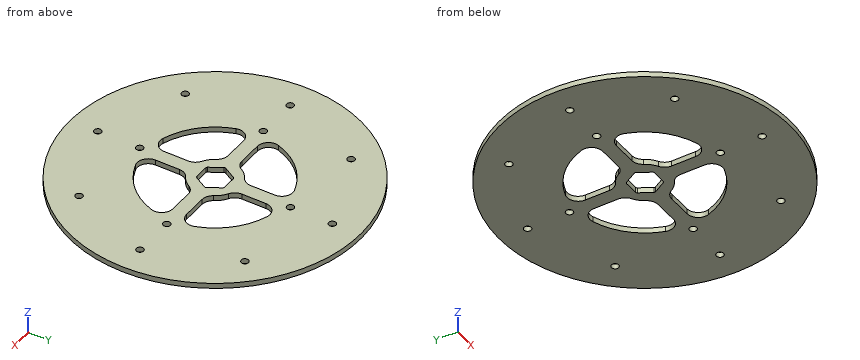
```python
from build123d import *

# Parameters (mm, degrees)
SKETCH1_R           = 66.548
SKETCH1_R_2         = 1.651
BOSS_EXTRUDE1_DEPTH = 2.4384
FILLET6_R           = 0.762


with BuildPart() as part:
    # Sketch1 → Boss-Extrude1 (new body)
    with BuildSketch(Plane.XY):
        Circle(SKETCH1_R)
        with Locations((0, 53.848)):
            Circle(SKETCH1_R_2, mode=Mode.SUBTRACT)
        with Locations((0, 34.619591715)):
            Circle(SKETCH1_R_2, mode=Mode.SUBTRACT)
        with Locations((34.619591715, 0)):
            Circle(SKETCH1_R_2, mode=Mode.SUBTRACT)
        with Locations((0, -34.619591715)):
            Circle(SKETCH1_R_2, mode=Mode.SUBTRACT)
        with Locations((-34.619591715, 0)):
            Circle(SKETCH1_R_2, mode=Mode.SUBTRACT)
        with Locations((38.076285953, 38.076285953)):
            Circle(SKETCH1_R_2, mode=Mode.SUBTRACT)
        with Locations((53.848, 0)):
            Circle(SKETCH1_R_2, mode=Mode.SUBTRACT)
        with Locations((38.076285953, -38.076285953)):
            Circle(SKETCH1_R_2, mode=Mode.SUBTRACT)
        with Locations((0, -53.848)):
            Circle(SKETCH1_R_2, mode=Mode.SUBTRACT)
        with Locations((-38.076285953, -38.076285953)):
            Circle(SKETCH1_R_2, mode=Mode.SUBTRACT)
        with Locations((-53.848, 0)):
            Circle(SKETCH1_R_2, mode=Mode.SUBTRACT)
        with Locations((-38.076285953, 38.076285953)):
            Circle(SKETCH1_R_2, mode=Mode.SUBTRACT)
        with BuildLine():
            Line((25.360281446, 3.175), (14.298079416, 3.175))
            ThreePointArc((14.298079416, 3.175), (11.758079416, 3.855590949), (9.898670365, 5.715))
            ThreePointArc((9.898670365, 5.715), (8.082230509, 8.082230509), (5.715, 9.898670365))
            ThreePointArc((5.715, 9.898670365), (3.855590949, 11.758079416), (3.175, 14.298079416))
            Line((3.175, 14.298079416), (3.175, 25.360281446))
            ThreePointArc((3.175, 25.360281446), (5.270146171, 29.470883302), (9.827380952, 30.190811245))
            ThreePointArc((9.827380952, 30.190811245), (22.450640303, 22.450640303), (30.190811245, 9.827380952))
            ThreePointArc((30.190811245, 9.827380952), (29.470883302, 5.270146171), (25.360281446, 3.175))
        make_face(mode=Mode.SUBTRACT)
        with BuildLine():
            Line((-3.175, 25.360281446), (-3.175, 14.298079416))
            ThreePointArc((-3.175, 14.298079416), (-3.855590949, 11.758079416), (-5.715, 9.898670365))
            ThreePointArc((-5.715, 9.898670365), (-8.082230509, 8.082230509), (-9.898670365, 5.715))
            ThreePointArc((-9.898670365, 5.715), (-11.758079416, 3.855590949), (-14.298079416, 3.175))
            Line((-14.298079416, 3.175), (-25.360281446, 3.175))
            ThreePointArc((-25.360281446, 3.175), (-29.470883302, 5.270146171), (-30.190811245, 9.827380952))
            ThreePointArc((-30.190811245, 9.827380952), (-22.450640303, 22.450640303), (-9.827380952, 30.190811245))
            ThreePointArc((-9.827380952, 30.190811245), (-5.270146171, 29.470883302), (-3.175, 25.360281446))
        make_face(mode=Mode.SUBTRACT)
        with BuildLine():
            Line((3.175, -25.360281446), (3.175, -14.298079416))
            ThreePointArc((3.175, -14.298079416), (3.855590949, -11.758079416), (5.715, -9.898670365))
            ThreePointArc((5.715, -9.898670365), (8.082230509, -8.082230509), (9.898670365, -5.715))
            ThreePointArc((9.898670365, -5.715), (11.758079416, -3.855590949), (14.298079416, -3.175))
            Line((14.298079416, -3.175), (25.360281446, -3.175))
            ThreePointArc((25.360281446, -3.175), (29.470883302, -5.270146171), (30.190811245, -9.827380952))
            ThreePointArc((30.190811245, -9.827380952), (22.450640303, -22.450640303), (9.827380952, -30.190811245))
            ThreePointArc((9.827380952, -30.190811245), (5.270146171, -29.470883302), (3.175, -25.360281446))
        make_face(mode=Mode.SUBTRACT)
        Polygon((7.332348419, 0), (3.666174209, 6.35), (-3.666174209, 6.35), (-7.332348419, 0), (-3.666174209, -6.35), (3.666174209, -6.35), align=None, mode=Mode.SUBTRACT)
        with BuildLine():
            Line((-25.360281446, -3.175), (-14.298079416, -3.175))
            ThreePointArc((-14.298079416, -3.175), (-11.758079416, -3.855590949), (-9.898670365, -5.715))
            ThreePointArc((-9.898670365, -5.715), (-8.082230509, -8.082230509), (-5.715, -9.898670365))
            ThreePointArc((-5.715, -9.898670365), (-3.855590949, -11.758079416), (-3.175, -14.298079416))
            Line((-3.175, -14.298079416), (-3.175, -25.360281446))
            ThreePointArc((-3.175, -25.360281446), (-5.270146171, -29.470883302), (-9.827380952, -30.190811245))
            ThreePointArc((-9.827380952, -30.190811245), (-22.450640303, -22.450640303), (-30.190811245, -9.827380952))
            ThreePointArc((-30.190811245, -9.827380952), (-29.470883302, -5.270146171), (-25.360281446, -3.175))
        make_face(mode=Mode.SUBTRACT)
    extrude(amount=BOSS_EXTRUDE1_DEPTH)

    # Fillet6
    fillet6_edges = [part.edges().sort_by_distance(p)[0] for p in [
        (3.666174209, -6.35, 1.2192),
        (7.332348419, 0, 1.2192),
        (3.666174209, 6.35, 1.2192),
        (-3.666174209, 6.35, 1.2192),
        (-7.332348419, 0, 1.2192),
        (-3.666174209, -6.35, 1.2192),
    ]]
    fillet(fillet6_edges, radius=FILLET6_R)


solid = part.part
```
CAD build for the part. Positions are in the model's coordinates, mm. Give positions to 0.01 mm unless a question says otherwise; leave off trailing zeros. Order: outer loops, then holes, each group sorted by start corner. A loop starts at its lowest first (then second) coordinate and runs counter-clockwise, first axis right, second up. Notation, with made-up numbers: M 17.25,35.25 L 34.25,35.25 A17 ccw 34.25,40.25 Z; hole C -23.75,5.5 d8. An arc over 180 degrees is marked long. Put each result on its own line as item: value. Start each with the question number.
(1) Saw through at A-A, the plane x = 0. Write the cut outline in (y, z), then the cut area to 3 significant figures.
(2) Drill centre lines: line 1 along Y through (x, z) = (0, 1); line 2 along Y through (x, z) = (10, 2.15); line 3 along Y through (x, z) = (-7.5, 1.1). Where is each one in solid material? Low to high.
(3) Saw through at B-B, the plane x = -22.5. Write the cut outline in (y, z) (3 decimals), then the cut area to 3 significant figures.
(4) Saw through at D-D, the plane y = -47.5. Write the cut outline in (x, z), then the cut area to 3 significant figures.
(5) Flat gauge pins, fed straight in: pin 1 Ø0.7 at (x, z) = (17.5, 1) entering from +Y; pin 2 Ø1.2 at (y, z) = (19.5, 1) entering from -X; pin 3 Ø1.2 at (y, z) = (18.5, 1.5) entering from +X. Where does each tip first touch, or does it go through?
(6) Saw through at C-C, the plane z = 0.5. Give the number of separate pieces and of enclosed holes in the cut face, then the cut area to 3 significant figures.
Check result:
1. outline: M -66.55,0 L -55.5,0 L -55.5,2.44 L -66.55,2.44 Z; M -52.2,0 L -36.27,0 L -36.27,2.44 L -52.2,2.44 Z; M -32.97,0 L -6.35,0 L -6.35,2.44 L -32.97,2.44 Z; M 6.35,0 L 32.97,0 L 32.97,2.44 L 6.35,2.44 Z; M 36.27,0 L 52.2,0 L 52.2,2.44 L 36.27,2.44 Z; M 55.5,0 L 66.55,0 L 66.55,2.44 L 55.5,2.44 Z
1. area: 261 mm2
2. line 1: y = -66.55 to -55.5, -52.2 to -36.27, -32.97 to -6.35, 6.35 to 32.97, 36.27 to 52.2, 55.5 to 66.55
2. line 2: y = -65.79 to -30.13, -5.55 to 5.55, 30.13 to 65.79
2. line 3: y = -66.12 to -30.38, -8.63 to 8.63, 30.38 to 66.12
3. outline: M -62.629,0 L -22.401,0 L -22.401,2.438 L -62.629,2.438 Z; M -3.175,0 L 3.175,0 L 3.175,2.438 L -3.175,2.438 Z; M 22.401,0 L 62.629,0 L 62.629,2.438 L 22.401,2.438 Z
3. area: 212 mm2
4. outline: M -46.61,0 L 46.61,0 L 46.61,2.44 L -46.61,2.44 Z
4. area: 227 mm2
5. pin 1: stops at y = 64.3
5. pin 2: stops at x = -63.81
5. pin 3: stops at x = 64.1
6. separate pieces: 1
6. enclosed holes: 17
6. area: 11,500 mm2
